from build123d import *

# Parameters (mm, degrees)
BOSS_EXTRUDE1_DEPTH = 5.8


with BuildPart() as part:
    # Sketch1 → Boss-Extrude1 (new body)
    with BuildSketch(Plane.XY):
        with BuildLine():
            Line((640.899853243, 447.602981641), (645.899853243, 447.602981641))
            ThreePointArc((645.899853243, 447.602981641), (648.899853243, 444.602981641), (645.899853243, 441.602981641))
            Line((645.899853243, 441.602981641), (640.899853243, 441.602981641))
            ThreePointArc((640.899853243, 441.602981641), (635.71651299, 433.661076237), (633.899853243, 424.352981641))
            Line((633.899853243, 424.352981641), (629.732441047, 424.352981641))
            Line((629.732441047, 424.352981641), (629.732441047, 428.928887757))
            Line((629.732441047, 428.928887757), (630.944771309, 428.928887757))
            Line((630.944771309, 428.928887757), (630.942520898, 431.328937702))
            Line((630.942520898, 431.328937702), (629.664733055, 431.349424729))
            Line((629.664733055, 431.349424729), (629.688208222, 432.81358455))
            Line((629.688208222, 432.81358455), (626.946903544, 432.857536436))
            Line((626.946903544, 432.857536436), (626.923428377, 431.393376615))
            Line((626.923428377, 431.393376615), (625.548423101, 431.415422349))
            Line((625.548423101, 431.415422349), (625.550673512, 429.015372404))
            Line((625.550673512, 429.015372404), (626.988308144, 429.015372404))
            Line((626.988308144, 429.015372404), (626.988308144, 424.439466289))
            Line((626.988308144, 424.439466289), (624.888308144, 424.439466289))
            Line((624.888308144, 424.439466289), (624.888308144, 418.439466289))
            Line((624.888308144, 418.439466289), (621.288308144, 418.439466289))
            Line((621.288308144, 418.439466289), (621.288308144, 424.439466289))
            Line((621.288308144, 424.439466289), (621.288308144, 464.766496994))
            Line((621.288308144, 464.766496994), (621.288308144, 470.766496994))
            Line((621.288308144, 470.766496994), (624.888308144, 470.766496994))
            Line((624.888308144, 470.766496994), (624.888308144, 464.766496994))
            Line((624.888308144, 464.766496994), (626.988308144, 464.766496994))
            Line((626.988308144, 464.766496994), (626.988308144, 460.190590879))
            Line((626.988308144, 460.190590879), (625.550673512, 460.190590879))
            Line((625.550673512, 460.190590879), (625.548423101, 457.790540934))
            Line((625.548423101, 457.790540934), (626.923428377, 457.812586668))
            Line((626.923428377, 457.812586668), (626.946903544, 456.348426847))
            Line((626.946903544, 456.348426847), (629.688208222, 456.392378732))
            Line((629.688208222, 456.392378732), (629.664733055, 457.856538553))
            Line((629.664733055, 457.856538553), (630.942520898, 457.877025581))
            Line((630.942520898, 457.877025581), (630.944771309, 460.277075526))
            Line((630.944771309, 460.277075526), (629.732441047, 460.277075526))
            Line((629.732441047, 460.277075526), (629.732441047, 464.852981641))
            Line((629.732441047, 464.852981641), (633.899853243, 464.852981641))
            ThreePointArc((633.899853243, 464.852981641), (635.71651299, 455.544887046), (640.899853243, 447.602981641))
        make_face()
    extrude(amount=BOSS_EXTRUDE1_DEPTH)


solid = part.part
Can you work these out from the model? Positions are in its coordinate system, mm. A direction names the side the tool comes from. Round coordinates to 2 decimals unless told otherwise and drop trailing zeros. Write each loop counter-clockwise with the first axis right and the second up, starting at its lowest first coordinate (ties: lowest second). Pieces come first, ordered by that corner, then holes. Notation, with made-up numbers: M 87.5,70.5 L 118.5,70.5 A14 ccw 118.5,97.5 Z; hole C -26.75,-2 d7. An arc over 180 degrees is marked long. Use a Markdown table: item, result.
Item 1: I want a section at D-D (y = 434). List the corners of the cut face in (x, z) for me, and give its area (3 significant figures).
Found:
| item | result |
|---|---|
| outline | M 621.29,0 L 635.86,0 L 635.86,5.8 L 621.29,5.8 Z |
| area | 84.5 mm2 |
Item 2: I want a section at B-B (y = 425). List the corners of the cut face in (x, z) for me, and give its area (3 significant figures).
Found:
| item | result |
|---|---|
| outline | M 621.29,0 L 626.99,0 L 626.99,5.8 L 621.29,5.8 Z; M 629.73,0 L 633.91,0 L 633.91,5.8 L 629.73,5.8 Z |
| area | 57.3 mm2 |
Item 3: Which directions (+Z, -Z, +X, -X, +Y, -Y) give clear straight access to the entire face, cutting with the end or side of a thin tool? Please do faces 1 (the face through (643, 441.603, 3)), 2 (the face through (626.988, 427, 3)), 3 (the face through (643, 447.603, 3)).
Found:
| item | result |
|---|---|
| face 1 | +Z, -Z, +X, -Y |
| face 2 | +Z, -Z, -Y |
| face 3 | +Z, -Z, +X, +Y |
Item 4: If I drill on line 1 along Y through (x, z) = (626.25, 4.65); line 2 along Y through (x, z) = (643, 3.2); line 3 along Y through (x, z) = (629.5, 1), over which ranges is the centre line in solid material (lowest first)? Write a range as [from, to].
Found:
| item | result |
|---|---|
| line 1 | y = [424.44, 429.02], [431.4, 457.8], [460.19, 464.77] |
| line 2 | y = [441.6, 447.6] |
| line 3 | y = [432.82, 456.39] |
Item 5: I want a section at C-C (x = 632.5). List the corners of the cut face in (y, z) for me.
Found:
| item | result |
|---|---|
| outline | M 424.35,0 L 464.85,0 L 464.85,5.8 L 424.35,5.8 Z |
Item 6: I want a section at A-A (y = 463). List the corners of the cut face in (x, z) for me, and give its area (3 significant figures).
Found:
| item | result |
|---|---|
| outline | M 621.29,0 L 626.99,0 L 626.99,5.8 L 621.29,5.8 Z; M 629.73,0 L 633.97,0 L 633.97,5.8 L 629.73,5.8 Z |
| area | 57.6 mm2 |
Item 7: For pin 1 Ø1.5 at (x, z) = (632, 3) entering from -Y; pin 2 Ø3 at (y, z) = (435.5, 4.5) entering from +X; pin 3 Ø0.6 at (x, z) = (630.5, 2) entering from +Y, each with a flat end and sliding along its axis, tell me the tip position at first contact or that it passes through.
Found:
| item | result |
|---|---|
| pin 1 | stops at y = 424.35 |
| pin 2 | stops at x = 637.37 |
| pin 3 | stops at y = 464.85 |
